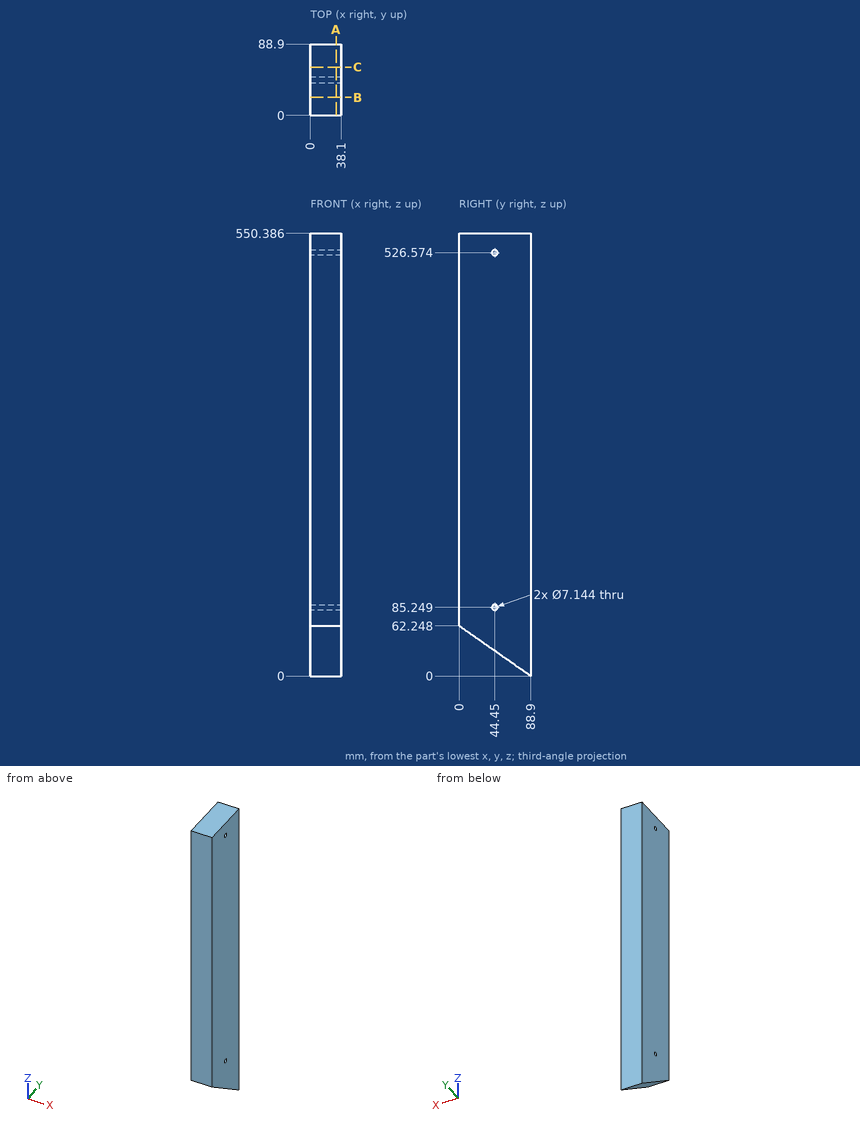
Answer from the drawing. Dimensions are ordinates in mm from the lowest x, y and z of the part. Give positions to 0.01 mm unless a question says otherwise; leave off trailing zeros. Order: outer loops, then holes, each group sorted by start corner. A loop starts at its lowest first (then second) coordinate and runs counter-clockwise, first axis right, second up. Notation, with made-up numbers: (-39.5, 57) -> (-3.5, 57) arc R22 cw to (-3.5, 64) -> close; hole circle Ø2 at (-14, 80.25). An arc over 180 degrees is marked (long way). One line per item, written item: value.
Item 1: Straight lines are drawn through the part: probe 1 along Z at (x, y) = (24, 30) (1 decimal); probe 2 along Z at (x, y) = (17, 33.5) (1 decimal); probe 3 along Y at (x, z) = (4, 60). For each, find the intervals that lie inside material, in ascending order.
Answer sheet:
probe 1: 41.2 to 550.4
probe 2: 38.8 to 550.4
probe 3: 3.21 to 88.9
Item 2: Find section B-B, the plane y = 22.5. Give the vertices of the cut face in (x, z), plus the area to 3 significant figures.
Answer sheet:
outline: (0, 46.49) -> (38.1, 46.49) -> (38.1, 550.39) -> (0, 550.39) -> close
area: 19,200 mm²
Item 3: Find section A-A, the plane x = 32. Give the vertices of the cut face in (y, z).
Answer sheet:
outline: (0, 62.25) -> (88.9, 0) -> (88.9, 550.39) -> (0, 550.39) -> close; hole circle Ø7.14 at (44.45, 85.25); hole circle Ø7.14 at (44.45, 526.57)
Item 4: Find section C-C, the plane y = 60. Give the vertices of the cut face in (x, z).
Answer sheet:
outline: (0, 20.24) -> (38.1, 20.24) -> (38.1, 550.39) -> (0, 550.39) -> close
Item 5: Flat-ended cylindrical pins translate along their axes: P1, Ø12, axis at x = 31.5, y = 29, coming from the -Z side; P2, Ø12, axis at y = 13, z = 460.5, coming from the -X side; P3, Ø6.5, axis at y = 44.45, z = 85.25, coming from the -X side. Find the tip coordinate at first contact, or state that the pin passes through.
Answer sheet:
P1: z = 37.74
P2: x = 0
P3: through
